Autodesk Inventor part; units mm, degrees
ref_plane "YZ Plane" through (0, 0, 0) normal (1, 0, 0) x (0, 1, 0)
ref_plane "XZ Plane" through (0, 0, 0) normal (0, 1, 0) x (-1, 0, 0)
ref_plane "XY Plane" through (0, 0, 0) normal (0, 0, 1) x (1, 0, 0)
sketch "Sketch1" plane through (0, 0, 0) normal (0, 0, 1) x (1, 0, 0)
  line L0 (-72.8091, 16.3486) -> (-72.8091, -13.2514)
  line L1 (-72.8091, -13.2514) -> (73.1909, -13.2514)
  line L2 (73.1909, -13.2514) -> (73.1909, 16.3486)
  line L3 (-72.8091, 16.3486) -> (-72.8091, 50.3486)
  line L4 (-72.8091, 50.3486) -> (73.1909, 50.3486)
  line L5 (73.1909, 50.3486) -> (73.1909, 16.3486)
  point P0 (0, 0)
  dimension "d0" = 34
extrude "Extrusion1" add sketch "Sketch1" along normal blind 6
sketch "Sketch2" plane through (0, 0, 6) normal (0, 0, 1) x (1, 0, 0)
  circle A0 centre (35, -5.2514) radius 3
  circle A1 centre (60, 9.7486) radius 3
  line L0 (0, 0) -> (0, 8.3537) construction
  circle A2 centre (-35, -5.2514) radius 3
  circle A3 centre (-60, 9.7486) radius 3
  line L1 (-72.8091, -13.2514) -> (73.1909, -13.2514)
  dimension "d3" = 6
  dimension "d4" = 6
  dimension "d6" = 15
  dimension "d7" = 60
  dimension "d10" = 8
  dimension "d11" = 35
extrude "Extrusion2" cut sketch "Sketch2" against normal through all
sketch "Sketch3" plane through (0, 0, 6) normal (0, 0, 1) x (1, 0, 0)
  circle A0 centre (2.1259, 1.3506) radius 2.25
  circle A1 centre (-15.3355, 11.1025) radius 2.25
  circle A2 centre (-15.6209, 31.1004) radius 2.25
  circle A3 centre (1.5552, 41.3465) radius 2.25
  circle A4 centre (19.0166, 31.5947) radius 2.25
  circle A5 centre (19.302, 11.5967) radius 2.25
  circle A6 centre (1.8405, 21.3486) radius 15 construction
  circle A7 centre (1.8405, 21.3486) radius 15.5
  point P0 (0, 0)
extrude "Extrusion3" cut sketch "Sketch3" against normal through all
sketch "Sketch5" plane through (0, 0, 0) normal (0, 0, -1) x (-1, 0, 0)
  line L0 (-73.1909, 16.3486) -> (-40.1909, 16.3486)
  line L1 (42.9091, 16.3486) -> (72.8091, 16.3486)
  circle A0 centre (-1.8405, 21.3486) radius 25 construction
  line L2 (-40.1909, 16.3486) -> (-26.3354, 16.3486)
  line L3 (42.9091, 16.3486) -> (22.6544, 16.3486)
  arc A1 (22.6544, 16.3486) -> (-26.3354, 16.3486) centre (-1.8405, 21.3486) ccw
  line L4 (-73.1909, 50.3486) -> (72.8091, 50.3486)
  line L5 (-73.1909, 50.3486) -> (72.8091, 50.3486)
  line L6 (72.8091, 16.3486) -> (72.8091, 50.3486)
  line L7 (-73.1909, 50.3486) -> (-73.1909, 16.3486)
  line L8 (-73.1909, -13.2514) -> (-73.1909, 50.3486)
  point P0 (0, 0)
extrude "Extrusion4" cut sketch "Sketch5" against normal through all
fillet "Fillet2" radius 40 2 edges at (-22.6544, 16.3486, 3) (26.3354, 16.3486, 3)
properties part number "x axis nut support"
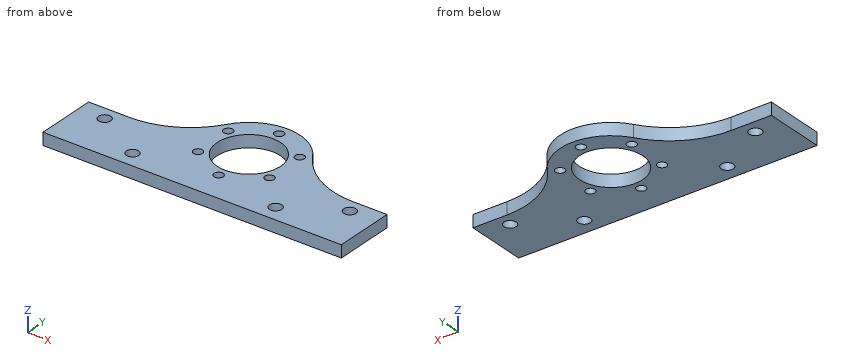
Work out the finished part from the listing and answer in its coordinate system (mm). Give positions to 0.01 mm unless a question says otherwise; leave off trailing zeros. Order: outer loops, then holes, each group sorted by start corner. A loop starts at its lowest first (then second) coordinate and runs counter-clockwise, first axis right, second up. Notation, with made-up numbers: (33.5, 61) -> (71.5, 61) arc R26 cw to (71.5, 100) -> close; hole circle Ø9 at (-32, 85.25). An arc over 180 degrees is marked (long way). Answer as CSV lines item,"result". Start each with the question number.
(1) Section D-D, the plane x = -24.5 is taken. Write down the section's boundary in (y, z), plus the area to 3 significant figures.
(2) Section C-C, the plane z = 2.2 is taken. Give the number of separate pieces and of enclosed holes in the cut face, plus the area to 3 significant figures.
(3) Each of these flat-tipped pins is pushed along its axis until it touches: pin 1 Ø2 at (x, z) = (20.5, 4) entering from +Y; pin 2 Ø5.5 at (x, y) = (-35, -5.25) entering from +Z; pin 3 Ø1 at (x, z) = (23, 1.5) entering from +Y. Where does it stop, or does it pass through?
(4) Section A-A, the plane x = -60 is taken. Write down the section's boundary in (y, z).
(5) Section B-B, the plane y = 26 is taken. Write down the section's boundary in (x, z).
(6) Consider line 1 along Y through (x, z) = (-16.5, 3.7); line 2 along Y through (x, z) = (1, 2.9); line 3 along Y through (x, z) = (4, 0.7). Determine where each line is inside the solid, lowest interval first.
Entries:
1,outline,"(-13.25, 0) -> (28.21, 0) -> (28.21, 6) -> (-13.25, 6) -> close"
1,area,"249 mm²"
2,separate pieces,"1"
2,enclosed holes,"11"
2,area,"4,850 mm²"
3,pin 1,"y = 39.04"
3,pin 2,"through"
3,pin 3,"y = 35.43"
4,outline,"(-13.25, 0) -> (6.75, 0) -> (6.75, 6) -> (-13.25, 6) -> close; (12.75, 0) -> (16.35, 0) -> (16.35, 6) -> (12.75, 6) -> close"
5,outline,"(-26.87, 0) -> (-12.95, 0) -> (-12.95, 6) -> (-26.87, 6) -> close; (16.63, 0) -> (30.56, 0) -> (30.56, 6) -> (16.63, 6) -> close"
6,line 1,"-13.25 to 9.18, 13.03 to 29.03, 33.17 to 38.34"
6,line 2,"-13.25 to -0.6, 3.3 to 5.87, 36.83 to 39.17, 43.53 to 46.33"
6,line 3,"-13.25 to 0.11, 2.6 to 6, 36.7 to 46.26"
